```python
from build123d import *

# Parameters (mm, degrees)
F0_R     = 11.9611676369
F1_DEPTH = 6.35


# Not quite as in the source:
# - a feature names something its author has since deleted; it is built from what else it names


with BuildPart() as f1:
    # F0 (on Top) → F1 (new body)
    with BuildSketch(Plane.XY):
        Polygon((4.9436837435, 38.7340840895), (-45.8563162565, 38.7340840895), (-45.8563162565, -50.1659159105), (55.7436837435, -50.1659159105), (55.7436837435, 38.7340840895), align=None)
        with Locations((30.3436837435, -5.7159159105)):
            Circle(F0_R, mode=Mode.SUBTRACT)
    extrude(amount=F1_DEPTH)


solid = f1.part
```
Read the model definition and answer for the solid it produces. Units are mm, in the model's axes. Round coordinates to 2 decimals unless told otherwise and drop trailing zeros. Write each loop counter-clockwise with the first axis right and the second up, starting at its lowest first coordinate (ties: lowest second). Pieces come first, ordered by that corner, then holes. Notation, with made-up numbers: (14.5, 2.25) -> (44.5, 2.25) arc R23 cw to (44.5, 17.25) -> close; hole circle Ø3 at (-15, 53). An arc over 180 degrees is marked (long way). Answer in a Markdown table with one row per item. Add a question column.
1) Determine the mould class of faces 1 (the face through (4, -5, 0)), 2 (the face through (6, 38.734, 3)), 3 (the face through (18.394, -5.19, 3.131)) for opening direction Y: pulls with the +Y half, pulls with the -Y half, needs draft (parallel to the pull), parting line crosses it, or undercut.
2) Find section A-A, the plane x = 28. Determine the outline of the cut face in (y, z).
3) Consider line 1 (X direction, y = -5, z = 5); line 2 (X direction, y = -10, z = 4.25); line 3 (Y direction, x = 23, z = 0.5). Determine where each line is inside the solid, lowest interval first.
4) Find section B-B, the plane y = -16.5. Determine the outline of the cut face in (x, z).
5) Find section C-C, the plane z = 2.5. Determine the outline of the cut face in (x, y), and give its area (3 significant figures).
Findings below:
| question | item | result |
|---|---|---|
| 1 | face 1 | needs draft |
| 1 | face 2 | pulls with the +Y half |
| 1 | face 3 | undercut |
| 2 | outline | (-50.17, 0) -> (-17.45, 0) -> (-17.45, 6.35) -> (-50.17, 6.35) -> close; (6.01, 0) -> (38.73, 0) -> (38.73, 6.35) -> (6.01, 6.35) -> close |
| 3 | line 1 | -45.86 to 18.4, 42.28 to 55.74 |
| 3 | line 2 | -45.86 to 19.18, 41.51 to 55.74 |
| 3 | line 3 | -50.17 to -15.16, 3.73 to 38.73 |
| 4 | outline | (-45.86, 0) -> (25.17, 0) -> (25.17, 6.35) -> (-45.86, 6.35) -> close; (35.52, 0) -> (55.74, 0) -> (55.74, 6.35) -> (35.52, 6.35) -> close |
| 5 | outline | (-45.86, -50.17) -> (55.74, -50.17) -> (55.74, 38.73) -> (-45.86, 38.73) -> close; hole circle Ø23.92 at (30.34, -5.72) |
| 5 | area | 8,580 mm² |
